Source: CAD feature listing. Evaluate the final solid. Frame: model axes, mm. Round coordinates to 2 decimals unless told otherwise and drop trailing zeros. Loops run counter-clockwise (first coordinate to the right, second up) from the corner with the lowest first, then second, coordinate; pieces in that order, holes last. Notation, with made-up numbers: M 12,-15 L 40,-15 A21 ccw 40,15 Z; hole C 78.5,35.25 d11. An arc over 180 degrees is marked long. Write each question's results on one line, items separated by ' | '. Start each with the question number.
1. Section A-A on x = 0. Output: boundary loops of the cut face in (y, z), and give its area (3 significant figures).
2. Contact query for flat-ended pins moving along their axis: pin 1 Ø8 at (x, z) = (92, 1030) entering from -Y; pin 2 Ø6 at (x, y) = (-16, 91.5) entering from +Z; pin 3 Ø12 at (x, z) = (-9.5, 1817.5) entering from +Y. Output: stop coordinate, or through.
3. Section C-C on y = 130. Output: boundary loops of the cut face in (x, z).
4. Ray query, line 1 (Y direction, x = 32, z = 150); line 2 (X direction, y = -57, z = 228); line 3 (Z direction, x = -108.5, y = 90). Return the intervals inside material, ascending.
5. Section B-B on z = 2261. Output: boundary loops of the cut face in (x, y).
from build123d import *

# Parameters (mm, degrees)
SKETCH1_R           = 152.4
BOSS_EXTRUDE1_DEPTH = 2494.28
CUT_EXTRUDE1_DEPTH  = 203.2
CUT_EXTRUDE2_DEPTH  = 203.2
FILLET1_R           = 152.4


with BuildPart() as part:
    # Sketch1 → Boss-Extrude1 (new body)
    with BuildSketch(Plane.XY):
        with Locations(Location((0, 0, 0), (0, 0, 180))):
            Circle(SKETCH1_R)
    extrude(amount=BOSS_EXTRUDE1_DEPTH)

    # Sketch3 → Cut-Extrude1 (cut, symmetric)
    with BuildSketch(Plane(origin=(0, 0, 0), x_dir=(0, 0, -1), z_dir=(1, 0, 0))):
        Polygon((-2361.35850174, 152.4), (-2494.28, 37.727132557), (-2330.25519021, -152.4), (-2701.978592606, -152.4), (-2701.978592606, 152.4), align=None)
    extrude(amount=CUT_EXTRUDE1_DEPTH, both=True, mode=Mode.SUBTRACT)

    # Sketch4 → Cut-Extrude2 (cut, symmetric)
    with BuildSketch(Plane(origin=(0, 0, 0), x_dir=(1, 0, 0), z_dir=(0, 1, 0))):
        with BuildLine():
            Line((-274.668681528, -2288.432323773), (-274.668681528, -2617.629818427))
            Line((-274.668681528, -2617.629818427), (274.668681528, -2617.629818427))
            Line((274.668681528, -2617.629818427), (274.668681528, -2288.432323773))
            Line((274.668681528, -2288.432323773), (152.4, -2288.432323773))
            add(Edge.make_bspline(
                [(152.4, -2288.432323773), (152.4, -2456.068889623), (76.2, -2494.28)],
                knots=[0, 0, 0, 1, 1, 1], degree=2, weights=[1, 0.380231012, 1]))
            Line((76.2, -2494.28), (-76.2, -2494.28))
            add(Edge.make_bspline(
                [(-152.4, -2288.432323773), (-152.4, -2456.068889623), (-76.2, -2494.28)],
                knots=[0, 0, 0, 1, 1, 1], degree=2, weights=[1, 0.380231012, 1]))
            Line((-152.4, -2288.432323773), (-274.668681528, -2288.432323773))
        make_face()
    extrude(amount=CUT_EXTRUDE2_DEPTH, both=True, mode=Mode.SUBTRACT)

    # Fillet1
    fillet1_edges = [part.edges().sort_by_distance(p)[0] for p in [
        (152.4, 0, 0),
    ]]
    fillet(fillet1_edges, radius=FILLET1_R)


solid = part.part
Taken from the geometry:
1) outline: M -152.4,152.4 A152.4 ccw 152.4,152.4 L 152.4,2361.36 L 37.73,2494.28 L -152.4,2330.26 Z | area: 727,000 mm^2
2) pin 1: y = -124.43 | pin 2: z = 2435.43 | pin 3: y = 152.36
3) outline: M -79.53,152.4 A79.53 ccw 79.53,152.4 L 79.53,2387.32 L -79.53,2387.32 Z
4) line 1: -148.98 to 148.98 | line 2: -141.34 to 141.34 | line 3: 94.49 to 2433.69
5) outline: C 0,0 d304.8
